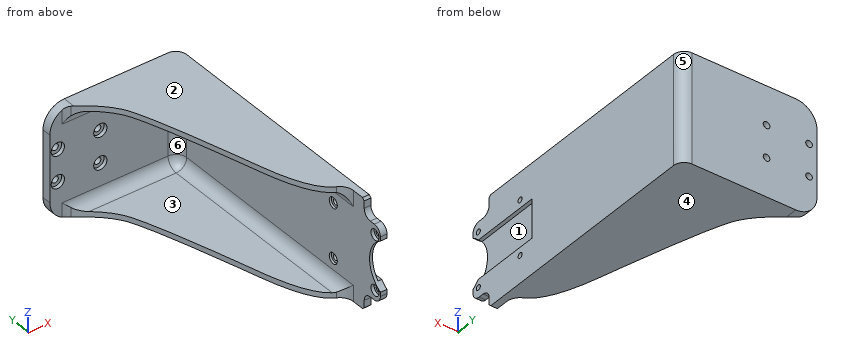
from build123d import *

# Parameters (mm, degrees)
SKETCH_1_W          = 51
SKETCH_1_H          = 41
SKETCH_1_R          = 1.25
EXTRUDE_1_DEPTH     = 3.4
SKETCH_2_R          = 1
EXTRUDE_2_DEPTH     = 2.5
SKETCH_3_W          = 14.5
SKETCH_3_H          = 35.737354226
CUT_EXTRUDE_1_DEPTH = 1.4
EXTRUDE_4_DEPTH     = 2
FILLET_1_R          = 8
FILLET_2_R          = 4
SKETCH_6_R          = 2
CUT_EXTRUDE_2_DEPTH = 1.2
CUT_EXTRUDE_3_DEPTH = 4
FILLET_3_R          = 3
SKETCH_9_R          = 2
CUT_EXTRUDE_4_DEPTH = 0.8
SKETCH_10_R         = 2.5
CUT_EXTRUDE_5_DEPTH = 1.4
CHAMFER_1_SIZE      = 0.8
FILLET_4_R          = 4
FILLET_5_R          = 5


with BuildPart() as part:
    # 草图1 → 凸台-拉伸1 (new body)
    with BuildSketch(Plane(origin=(0, 0, 0), x_dir=(1, 0, 0), z_dir=(0, 1, 0))):
        Rectangle(SKETCH_1_W, SKETCH_1_H)
        with Locations(Location((-22.5, 6, 0), (0, 0, 270))):
            Circle(SKETCH_1_R, mode=Mode.SUBTRACT)
        with Locations(Location((-22.5, -6, 0), (0, 0, 90))):
            Circle(SKETCH_1_R, mode=Mode.SUBTRACT)
        with Locations(Location((-6.5, 6, 0), (0, 0, 270))):
            Circle(SKETCH_1_R, mode=Mode.SUBTRACT)
        with Locations(Location((-6.5, -6, 0), (0, 0, 90))):
            Circle(SKETCH_1_R, mode=Mode.SUBTRACT)
    extrude(amount=EXTRUDE_1_DEPTH)

    # 草图2 → 凸台-拉伸2 (add)
    with BuildSketch(Plane(origin=(25.5, 0, 0), x_dir=(0, 0, -1), z_dir=(1, 0, 0))):
        with BuildLine():
            Line((-20.5, 0), (20.5, 0))
            Line((20.5, 0), (20.5, -100))
            Line((20.5, -100), (9.43808773, -100))
            ThreePointArc((9.43808773, -100), (0, -94.65), (-9.43808773, -100))
            Line((-9.43808773, -100), (-20.5, -100))
            Line((-20.5, -100), (-20.5, 0))
        make_face()
        with Locations((-10.25, -97.35)):
            Circle(SKETCH_2_R, mode=Mode.SUBTRACT)
        with Locations(Location((10.25, -97.35, 0), (0, 0, 180))):
            Circle(SKETCH_2_R, mode=Mode.SUBTRACT)
        with Locations((10.25, -76.65)):
            Circle(SKETCH_2_R, mode=Mode.SUBTRACT)
        with Locations(Location((-10.25, -76.65, 0), (0, 0, 180))):
            Circle(SKETCH_2_R, mode=Mode.SUBTRACT)
    extrude(amount=-EXTRUDE_2_DEPTH)

    # 草图3 → 切除-拉伸1 (cut)
    with BuildSketch(Plane(origin=(25.5, 0, 0), x_dir=(0, 0, -1), z_dir=(1, 0, 0))):
        with Locations((0, -88.518677113)):
            Rectangle(SKETCH_3_W, SKETCH_3_H)
    extrude(amount=-CUT_EXTRUDE_1_DEPTH, mode=Mode.SUBTRACT)

    # 草图5 → 凸台-拉伸4 (add)
    with BuildSketch(Plane(origin=(0, 0, -20.5), x_dir=(-1, 0, 0), z_dir=(0, 0, -1))):
        with BuildLine():
            Line((-25.5, 3.4), (19.5, 3.4))
            Line((19.5, 3.4), (19.5, 0))
            add(Edge.make_bspline(
                [(19.5, 0), (10.67122189, -5.3692624), (2.779429236, -18.193392293), (-14.23746955, -82.475470635), (-23, -82.805044976)],
                knots=[0, 0, 0, 0.396049025, 0.788579615, 1, 1, 1], degree=2))
            Line((-23, -82.805044976), (-25.5, -82.805044976))
            Line((-25.5, -82.805044976), (-25.5, 3.4))
        make_face()
    extrude_4 = extrude(amount=-EXTRUDE_4_DEPTH)

    # 镜向3: 凸台-拉伸4 across plane
    add(extrude_4.mirror(Plane.XY))

    # 圆角1
    fillet_1_edges = [part.edges().sort_by_distance(p)[0] for p in [
        (-25.5, 1.7, -20.5),
        (-25.5, 1.7, 20.5),
    ]]
    fillet(fillet_1_edges, radius=FILLET_1_R)

    # 圆角2
    fillet_2_edges = [part.edges().sort_by_distance(p)[0] for p in [
        (25.5, 3.4, 0),
        (23, 0, 0),
    ]]
    fillet(fillet_2_edges, radius=FILLET_2_R)

    # 草图6 → 切除-拉伸2 (cut)
    with BuildSketch(Plane.ZY.offset(-23)):
        with Locations((10.25, -97.35)):
            Circle(SKETCH_6_R)
        with Locations((-10.25, -97.35)):
            Circle(SKETCH_6_R)
    extrude(amount=-CUT_EXTRUDE_2_DEPTH, mode=Mode.SUBTRACT)

    # 草图8 → 切除-拉伸3 (cut)
    with BuildSketch(Plane(origin=(25.5, 0, 0), x_dir=(0, 0, -1), z_dir=(1, 0, 0))):
        Polygon((14, -102.818047241), (14, -92), (23.468492482, -92), (23.468492482, -110.008191191), (-23.468492482, -110.008191191), (-23.468492482, -92), (-14, -92), (-14, -102.818047241), align=None)
    extrude(amount=-CUT_EXTRUDE_3_DEPTH, mode=Mode.SUBTRACT)

    # 圆角3
    fillet_3_edges = [part.edges().sort_by_distance(p)[0] for p in [
        (24.25, -100, 14),
        (24.25, -100, -14),
        (24.25, -92, -14),
        (24.25, -92, 14),
    ]]
    fillet(fillet_3_edges, radius=FILLET_3_R)

    # 草图9 → 切除-拉伸4 (cut)
    with BuildSketch(Plane.ZY.offset(-23)):
        with Locations((10.25, -76.65)):
            Circle(SKETCH_9_R)
        with Locations(Location((-10.25, -76.65, 0), (0, 0, 180))):
            Circle(SKETCH_9_R)
    extrude(amount=-CUT_EXTRUDE_4_DEPTH, mode=Mode.SUBTRACT)

    # 草图10 → 切除-拉伸5 (cut)
    with BuildSketch(Plane(origin=(0, 0, 0), x_dir=(-1, 0, 0), z_dir=(0, -1, 0))):
        with Locations(Location((6.5, -6, 0), (0, 0, 90))):
            Circle(SKETCH_10_R)
        with Locations(Location((22.5, -6, 0), (0, 0, 270))):
            Circle(SKETCH_10_R)
        with Locations(Location((6.5, 6, 0), (0, 0, 270))):
            Circle(SKETCH_10_R)
        with Locations(Location((22.5, 6, 0), (0, 0, 90))):
            Circle(SKETCH_10_R)
    extrude(amount=-CUT_EXTRUDE_5_DEPTH, mode=Mode.SUBTRACT)

    # 倒角1
    chamfer_1_edges = [part.edges().sort_by_distance(p)[0] for p in [
        (24.25, -92, 20.5),
        (24.25, -92, -20.5),
    ]]
    chamfer(chamfer_1_edges, length=CHAMFER_1_SIZE)

    # 圆角4
    fillet_4_edges = [part.edges().sort_by_distance(p)[0] for p in [
        (-0.25, 0, -18.5),
        (21.828427125, -1.171572875, -18.5),
        (-0.25, 0, 18.5),
        (21.828427125, -1.171572875, 18.5),
        (23, -43.402522488, -18.5),
        (23, -43.402522488, 18.5),
    ]]
    fillet(fillet_4_edges, radius=FILLET_4_R)

    # 圆角5
    fillet_5_edges = [part.edges().sort_by_distance(p)[0] for p in [
        (23, -82.805044976, 16.5),
        (23, -82.805044976, -16.5),
        (-19.5, 0, 16.5),
        (-19.5, 0, -16.5),
    ]]
    fillet(fillet_5_edges, radius=FILLET_5_R)


solid = part.part
Source: CAD feature listing. Evaluate the final solid. Frame: model axes, mm. Face numbers are marked on the shaded views. A direction names the side the tool comes from. Give positions to 0.01 mm unless a question says otherwise; leave off trailing zeros. Write each loop counter-clockwise with the first axis right and the second up, starting at its lowest first coordinate (ties: lowest second). Pieces come first, ordered by that corner, then holes. Notation, with made-up numbers: M 70,10 L 82,10 A22 ccw 82,47 Z; hole C 24.25,23 d8. An arc over 180 degrees is marked long. Answer as a JSON object with one key per item and string values.
Q1. Ray query, line 1 along Y through (x, z) = (24.95, 10.25); line 2 along Z through (x, y) = (14, -51); line 3 along X through (y, z) = (1, -6). Return the intervals inside material, ascending.
Geometry check:
{"line 1": "y = -100 to -98.35, -96.35 to -77.65, -75.65 to 1.42", "line 2": "z = -20.5 to -18.5, 18.5 to 20.5", "line 3": "x = -25.5 to -25, -20 to -9, -4 to 25.17"}
Q2. Access query for the marked faces 1, 2 and 3. Directions: +Z, -Z, +X, -X, +Y, -Y. A direction counts if a zero-diameter tool reaches every point of the face in a straight line with its end or side. Return the directions, or none.
Geometry check:
{"face 1": "+X, -Y", "face 2": "+Z, +X, -X, +Y, -Y", "face 3": "-X, -Y"}
Q3. Cut plane A-A, the plane x = -22.5. Return the cut outline in (y, z) (3 decimals), then the cut area to 3 significant figures.
Geometry check:
{"outline": "M 0,-18.745 L 3.4,-18.745 L 3.4,-7.25 L 1.4,-7.25 L 1.4,-8.5 L 0,-8.5 Z; M 0,-3.5 L 1.4,-3.5 L 1.4,-4.75 L 3.4,-4.75 L 3.4,4.75 L 1.4,4.75 L 1.4,3.5 L 0,3.5 Z; M 0,8.5 L 1.4,8.5 L 1.4,7.25 L 3.4,7.25 L 3.4,18.745 L 0,18.745 Z", "area": "103 mm^2"}
Q4. Cut plane C-C, the plane x = -6.5. Count the separate pieces of the cut face and the enclosed holes in it, then the cut area to 3 significant figures.
Geometry check:
{"separate pieces": "3", "enclosed holes": "0", "area": "171 mm^2"}
Q5. Contact query for flat-ended pins moving along their axis: P1, Ø1.2, axis at y = -76, z = 10.5, coming from the -X side; P2, Ø3, axis at y = -97.35, z = 10.25, coming from the -X side; P3, Ø1.5, axis at x = -19, z = -13, coming from the -Y side. Output: stop coordinate, or through.
Geometry check:
{"P1": "stops at x = 23.8", "P2": "stops at x = 24.2", "P3": "stops at y = 0"}
Q6. Mould query, pull axis Z, two halves, no side actions, for the marked faces 4, 5 and 6. Classes: +Z half, -Z half, draft (parallel to the pull), parting line (faces both ways), or undercut.
Geometry check:
{"face 4": "-Z half", "face 5": "draft", "face 6": "undercut"}
Q7. Cut plane B-B, the plane z = -6. Return the cut outline in (x, y).
Geometry check:
{"outline": "M -25.5,0 L -25,0 L -25,1.4 L -23.75,1.4 L -23.75,3.4 L -25.5,3.4 Z; M -21.25,1.4 L -20,1.4 L -20,0 L -9,0 L -9,1.4 L -7.75,1.4 L -7.75,3.4 L -21.25,3.4 Z; M -5.25,1.4 L -4,1.4 L -4,0 L 19,0 A4 cw 23,-4 L 23,-96.43 L 24.1,-96.43 L 24.1,-70.65 L 25.5,-70.65 L 25.5,-0.6 A4 ccw 21.5,3.4 L -5.25,3.4 Z"}
